The listing builds one solid part. Answer for the finished solid, in the listing's coordinates (mm). A direction names the side the tool comes from. Give positions to 0.01 mm unless a question says otherwise; leave off trailing zeros. Order: outer loops, then holes, each group sorted by start corner. A loop starts at its lowest first (then second) coordinate and runs counter-clockwise, first axis right, second up. Notation, with made-up numbers: (59.5, -9.5) - (114.5, -9.5) arc R25 ccw to (114.5, 12.5) - close; hole circle Ø2 at (44, 87). An arc over 180 degrees is marked (long way). Answer as CSV lines item,"result". Start each with the question number.
1. Section C-C on x = -56.5 is taken. Give the vertices of the cut face in (y, z).
2. Section B-B on z = 46 is taken. Give the vertices of the cut face in (x, y).
3. Section A-A on y = 21 is taken. Give the vertices of the cut face in (x, z).
4. Which of the six approach directions +Z, -Z, +X, -X, +Y, -Y give full straight-line access (tool end or side, diameter ignored) to faces 4 (the flat face through (-1, 0, 25)), 5 (the flat face through (101.5, 20, 25)), 6 (the cylindrical face through (-108.93, 53.87, 35.25)), 7 (the flat face through (-109, 49, 25))?
5. Consider line 1 along Z through (x, y) = (109, 55.75); line 2 along X through (y, z) = (52, 12.5); line 3 along X through (y, z) = (37, 38). Determine where each line is inside the solid, lowest interval first. Write a range as [from, to].
6. Flat-ended cylindrical pins translate along their axes: pin 1 (6 mm diameter, centred on x = -109, z = 12.5, fed in from -Y); pin 2 (25 mm diameter, centred on y = 29, z = 28.5, fed in from +X); pin 3 (25 mm diameter, centred on x = -30.5, z = 17, fed in from +Y). Find the tip coordinate at first contact, or state that the pin passes through.
7. Determine the mould class of faces 1 (the cylindrical face through (109.07, 53.87, 35.25)), 2 (the flat face through (-1, -4, 50)), 3 (the flat face through (93.5, 28, 25)) for opening direction Z: +Z half, -Z half, draft (parallel to the pull), parting line (faces both ways), or undercut.
Autodesk Fusion 360 part; units mm, degrees
sketch "Outline" plane through (0, 0, 0) normal (0, 0, 1) x (1, 0, 0)
  line L0 (0, 0) -> (0, 56.9537) construction
  line L1 (0, 0) -> (93.5, 0)
  line L2 (93.5, 0) -> (93.5, 57)
  line L3 (93.5, 57) -> (116.5, 57)
  line L4 (116.5, 57) -> (116.5, 49)
  line L5 (-93.5, 57) -> (-116.5, 57)
  line L6 (-93.5, 0) -> (-93.5, 57)
  line L7 (0, 0) -> (-93.5, 0)
  line L8 (-101.5, -8) -> (-101.5, 49)
  line L9 (-101.5, 49) -> (-116.5, 49)
  line L10 (-116.5, 57) -> (-116.5, 49)
  line L11 (101.5, -8) -> (101.5, 49)
  line L12 (101.5, 49) -> (116.5, 49)
  line L13 (-101.5, -8) -> (101.5, -8)
  dimension "d2" = 187
  dimension "d3" = 57
  dimension "d6" = 23
  dimension "d8" = 8
  dimension "d9" = 8
  dimension "d10" = 8
extrude "Extrude1" add sketch "Outline" along normal blind 50
sketch "Holes for Mounting" plane through (0, 49, 0) normal (0, -1, 0) x (1, 0, 0)
  line L0 (-116.5, 0) -> (-101.5, 0)
  line L1 (-101.5, 0) -> (-101.5, 50)
  line L2 (-101.5, 50) -> (-116.5, 50)
  line L3 (-116.5, 50) -> (-116.5, 0)
  line L4 (101.5, 0) -> (116.5, 0)
  line L5 (116.5, 0) -> (116.5, 50)
  line L6 (116.5, 50) -> (101.5, 50)
  line L7 (101.5, 50) -> (101.5, 0)
  line L8 (0, 0) -> (0, 29.5518) construction
  line L9 (-109, 50) -> (-109, 0) construction
  circle A0 centre (-109, 12.5) radius 4
  line L10 (-116.5, 25) -> (-101.5, 25) construction
  circle A1 centre (-109, 37.5) radius 4
  circle A2 centre (109, 12.5) radius 4
  circle A3 centre (109, 37.5) radius 4
  dimension "d13" = 25
  dimension "d14" = 8
hole "Hole1" at (-109, 49, 12.5) at (-109, 49, 37.5) at (109, 49, 12.5) at (109, 49, 37.5) direction (0, 1, 0) diameter 4.5 depth 15 tip angle 118 countersink diameter 7.8 countersink angle 90
sketch "Make those holes 3d printable" plane through (0, 49, 0) normal (0, -1, 0) x (1, 0, 0)
  circle A0 centre (-109, 37.5) radius 2.25
  circle A1 centre (-109, 12.5) radius 2.25
  circle A2 centre (-109, 12.5) radius 3.9
  circle A3 centre (-109, 37.5) radius 3.9
  line L0 (-116.5, 0) -> (-101.5, 0)
  line L1 (-101.5, 0) -> (-101.5, 50)
  line L2 (-101.5, 50) -> (-116.5, 50)
  line L3 (-116.5, 50) -> (-116.5, 0)
  circle A4 centre (109, 12.5) radius 2.25
  circle A5 centre (109, 12.5) radius 3.9
  circle A6 centre (109, 37.5) radius 3.9
  line L4 (101.5, 0) -> (116.5, 0)
  line L5 (116.5, 0) -> (116.5, 50)
  line L6 (116.5, 50) -> (101.5, 50)
  line L7 (101.5, 50) -> (101.5, 0)
  circle A7 centre (109, 37.5) radius 2.25
  line L8 (0, 0) -> (0, 31.3528) construction
  line L9 (-109, 12.5) -> (-109, 37.5) construction
  line L10 (-109, 15.682) -> (-107.409, 14.091)
  line L11 (-109, 15.682) -> (-110.591, 14.091)
  line L12 (-109, 37.5) -> (-109, 47.9653) construction
  line L13 (-109, 40.682) -> (-107.409, 39.091)
  line L14 (-109, 40.682) -> (-110.591, 39.091)
  line L15 (109, 40.682) -> (110.591, 39.091)
  line L16 (109, 40.682) -> (107.409, 39.091)
  line L17 (109, 15.682) -> (110.591, 14.091)
  line L18 (109, 15.682) -> (107.409, 14.091)
extrude "Extrude2" cut sketch "Make those holes 3d printable" against normal blind 8 contours A0 L13 L14 | A1 L10 L11 | A4 L17 L18 | A7 L15 L16
equation "d6 = 15 mm + 8 mm"
equation "d9 = d8"
equation "d10 = d8"
Checks:
1,outline,"(-8, 0) - (0, 0) - (0, 50) - (-8, 50) - close"
2,outline,"(-116.5, 49) - (-101.5, 49) - (-101.5, -8) - (101.5, -8) - (101.5, 49) - (116.5, 49) - (116.5, 57) - (93.5, 57) - (93.5, 0) - (-93.5, 0) - (-93.5, 57) - (-116.5, 57) - close"
3,outline,"(-101.5, 0) - (-93.5, 0) - (-93.5, 50) - (-101.5, 50) - close; (93.5, 0) - (101.5, 0) - (101.5, 50) - (93.5, 50) - close"
4,face 4,"+Z, -Z, +Y"
4,face 5,"+Z, -Z, +X, -Y"
4,face 6,"+Y, -Y"
4,face 7,"+Z, -Z, -X, -Y"
5,line 1,"z = [0, 10.25], [15.68, 35.25], [40.68, 50]"
5,line 2,"x = [-116.5, -111.25], [-106.75, -93.5], [93.5, 106.75], [111.25, 116.5]"
5,line 3,"x = [-101.5, -93.5], [93.5, 101.5]"
6,pin 1,"stops at y = 49.9"
6,pin 2,"stops at x = 101.5"
6,pin 3,"stops at y = 0"
7,face 1,"undercut"
7,face 2,"+Z half"
7,face 3,"draft"
